The listing builds one solid part. Answer for the finished solid, in the listing's coordinates (mm). Round coordinates to 2 decimals unless told otherwise and drop trailing zeros. Loops run counter-clockwise (first coordinate to the right, second up) from the corner with the lowest first, then second, coordinate; pieces in that order, holes last. Notation, with made-up numbers: (78.25, 40.5) -> (120.25, 40.5) arc R21 cw to (120.25, 51.5) -> close; hole circle Ø3 at (36, 74). An arc over 180 degrees is marked (long way). Write each question's results on one line, items separated by ' | '. Start each with the question number.
(1) The part is cut by section A-A (x = 63). Determine the outline of the cut face in (y, z), plus the area to 3 significant figures.
(2) Flat-ended cylindrical pins translate along their axes: pin 1 (0.9 mm diameter, centred on x = 118.5, y = 1.5, fed in from -Z); pin 2 (1.5 mm diameter, centred on x = 118, y = 2, fed in from +Z); pin 3 (1.5 mm diameter, centred on x = 118, y = 1.5, fed in from -Z). Find the tip coordinate at first contact, or state that the pin passes through.
(3) The part is cut by section B-B (z = -28). Determine the outline of the cut face in (x, y).
(4) The part is cut by section C-C (x = 102.5). Determine the outline of the cut face in (y, z).
(5) The part is cut by section D-D (y = 1.45). Count the separate pieces of the cut face and the enclosed holes in it, plus the area to 3 significant figures.
(6) Straight lines are drawn through the part: probe 1 along X at (y, z) = (1.85, -60); probe 2 along Z at (x, y) = (82.5, 2.15); probe 3 along Z at (x, y) = (67.5, 0.9). For each, find the intervals that lie inside material, in ascending order.
```python
from build123d import *

# Parameters (mm, degrees)
BOSS_EXTRUDE1_DEPTH = 3
CUT_EXTRUDE1_REACH  = 162.106
SKETCH2_W           = 45
SKETCH2_H           = 74
FILLET2_R           = 3
SKETCH3_W           = 3.1
SKETCH3_H           = 10.1
CUT_EXTRUDE2_DEPTH  = 161.106214745
CUT_EXTRUDE3_REACH  = 162.106
SKETCH4_R           = 1.6


with BuildPart() as part:
    # Sketch1 → Boss-Extrude1 (new body)
    with BuildSketch(Plane(origin=(0, 0, 0), x_dir=(1, 0, 0), z_dir=(0, 1, 0))):
        Polygon((42.5, 100), (85, 100), (125, 76.905989232), (125, -76.905989232), (85, -100), (42.5, -100), align=None)
        with BuildLine():
            Line((99.3, 23), (67.3, 23))
            ThreePointArc((67.3, 23), (63.764466094, 21.535533906), (62.3, 18))
            Line((62.3, 18), (62.3, -14))
            ThreePointArc((62.3, -14), (63.764466094, -17.535533906), (67.3, -19))
            Line((67.3, -19), (99.3, -19))
            ThreePointArc((99.3, -19), (102.835533906, -17.535533906), (104.3, -14))
            Line((104.3, -14), (104.3, 18))
            ThreePointArc((104.3, 18), (102.835533906, 21.535533906), (99.3, 23))
        make_face(mode=Mode.SUBTRACT)
    extrude(amount=BOSS_EXTRUDE1_DEPTH)

    # Sketch2 → Cut-Extrude1 (cut, up to next)
    with BuildSketch(Plane(origin=(0, 3, 0), x_dir=(1, 0, 0), z_dir=(0, 1, 0)), mode=Mode.PRIVATE) as cut_extrude1_sk1:
        with Locations((65, 18)):
            Rectangle(SKETCH2_W, SKETCH2_H)
    cut_extrude1_tool1 = extrude(cut_extrude1_sk1.sketch, amount=-CUT_EXTRUDE1_REACH, mode=Mode.PRIVATE) & part.part
    add(cut_extrude1_tool1.solids().sort_by_distance((65, 3, -18))[0], mode=Mode.SUBTRACT)

    # Fillet2
    fillet2_edges = [part.edges().sort_by_distance(p)[0] for p in [
        (125, 1.5, -76.905989232),
        (125, 1.5, 76.905989232),
        (85, 1.5, 100),
        (42.5, 1.5, 100),
        (42.5, 1.5, -100),
        (85, 1.5, -100),
        (42.5, 1.5, 19),
        (42.5, 1.5, -55),
        (87.5, 1.5, -23),
        (87.5, 1.5, -55),
    ]]
    fillet(fillet2_edges, radius=FILLET2_R)

    # Sketch3 → Cut-Extrude2 (cut, through all)
    with BuildSketch(Plane(origin=(0, 3, 0), x_dir=(1, 0, 0), z_dir=(0, 1, 0))):
        with Locations((118.45, 20)):
            Rectangle(SKETCH3_W, SKETCH3_H)
        with Locations((118.45, -20)):
            Rectangle(SKETCH3_W, SKETCH3_H)
        with Locations((118.45, 60)):
            Rectangle(SKETCH3_W, SKETCH3_H)
        with Locations((118.45, -60)):
            Rectangle(SKETCH3_W, SKETCH3_H)
    extrude(amount=-CUT_EXTRUDE2_DEPTH, mode=Mode.SUBTRACT)

    # Sketch4 → Cut-Extrude3 (cut, up to next)
    with BuildSketch(Plane(origin=(0, 3, 0), x_dir=(1, 0, 0), z_dir=(0, 1, 0)), mode=Mode.PRIVATE) as cut_extrude3_sk1:
        with Locations(Location((50.5, 92, 0), (0, 0, 270))):
            Circle(SKETCH4_R)
    cut_extrude3_tool1 = extrude(cut_extrude3_sk1.sketch, amount=-CUT_EXTRUDE3_REACH, mode=Mode.PRIVATE) & part.part
    # Sketch4 → Cut-Extrude3 (cut, up to next)
    with BuildSketch(Plane(origin=(0, 3, 0), x_dir=(1, 0, 0), z_dir=(0, 1, 0)), mode=Mode.PRIVATE) as cut_extrude3_sk2:
        with Locations(Location((47.5, 60, 0), (0, 0, 270))):
            Circle(SKETCH4_R)
    cut_extrude3_tool2 = extrude(cut_extrude3_sk2.sketch, amount=-CUT_EXTRUDE3_REACH, mode=Mode.PRIVATE) & part.part
    # Sketch4 → Cut-Extrude3 (cut, up to next)
    with BuildSketch(Plane(origin=(0, 3, 0), x_dir=(1, 0, 0), z_dir=(0, 1, 0)), mode=Mode.PRIVATE) as cut_extrude3_sk3:
        with Locations(Location((47.5, -60, 0), (0, 0, 270))):
            Circle(SKETCH4_R)
    cut_extrude3_tool3 = extrude(cut_extrude3_sk3.sketch, amount=-CUT_EXTRUDE3_REACH, mode=Mode.PRIVATE) & part.part
    # Sketch4 → Cut-Extrude3 (cut, up to next)
    with BuildSketch(Plane(origin=(0, 3, 0), x_dir=(1, 0, 0), z_dir=(0, 1, 0)), mode=Mode.PRIVATE) as cut_extrude3_sk4:
        with Locations(Location((50.5, -92, 0), (0, 0, 270))):
            Circle(SKETCH4_R)
    cut_extrude3_tool4 = extrude(cut_extrude3_sk4.sketch, amount=-CUT_EXTRUDE3_REACH, mode=Mode.PRIVATE) & part.part
    # Sketch4 → Cut-Extrude3 (cut, up to next)
    with BuildSketch(Plane(origin=(0, 3, 0), x_dir=(1, 0, 0), z_dir=(0, 1, 0)), mode=Mode.PRIVATE) as cut_extrude3_sk5:
        with Locations(Location((117, 72.287187079, 0), (0, 0, 270))):
            Circle(SKETCH4_R)
    cut_extrude3_tool5 = extrude(cut_extrude3_sk5.sketch, amount=-CUT_EXTRUDE3_REACH, mode=Mode.PRIVATE) & part.part
    # Sketch4 → Cut-Extrude3 (cut, up to next)
    with BuildSketch(Plane(origin=(0, 3, 0), x_dir=(1, 0, 0), z_dir=(0, 1, 0)), mode=Mode.PRIVATE) as cut_extrude3_sk6:
        with Locations(Location((117, -72.287187079, 0), (0, 0, 270))):
            Circle(SKETCH4_R)
    cut_extrude3_tool6 = extrude(cut_extrude3_sk6.sketch, amount=-CUT_EXTRUDE3_REACH, mode=Mode.PRIVATE) & part.part
    # Sketch4 → Cut-Extrude3 (cut, up to next)
    with BuildSketch(Plane(origin=(0, 3, 0), x_dir=(1, 0, 0), z_dir=(0, 1, 0)), mode=Mode.PRIVATE) as cut_extrude3_sk7:
        with Locations(Location((82.856406461, 92, 0), (0, 0, 270))):
            Circle(SKETCH4_R)
    cut_extrude3_tool7 = extrude(cut_extrude3_sk7.sketch, amount=-CUT_EXTRUDE3_REACH, mode=Mode.PRIVATE) & part.part
    # Sketch4 → Cut-Extrude3 (cut, up to next)
    with BuildSketch(Plane(origin=(0, 3, 0), x_dir=(1, 0, 0), z_dir=(0, 1, 0)), mode=Mode.PRIVATE) as cut_extrude3_sk8:
        with Locations(Location((82.856406461, -92, 0), (0, 0, 270))):
            Circle(SKETCH4_R)
    cut_extrude3_tool8 = extrude(cut_extrude3_sk8.sketch, amount=-CUT_EXTRUDE3_REACH, mode=Mode.PRIVATE) & part.part
    add(cut_extrude3_tool1.solids().sort_by_distance((50.5, 3, -92))[0], mode=Mode.SUBTRACT)
    add(cut_extrude3_tool2.solids().sort_by_distance((47.5, 3, -60))[0], mode=Mode.SUBTRACT)
    add(cut_extrude3_tool3.solids().sort_by_distance((47.5, 3, 60))[0], mode=Mode.SUBTRACT)
    add(cut_extrude3_tool4.solids().sort_by_distance((50.5, 3, 92))[0], mode=Mode.SUBTRACT)
    add(cut_extrude3_tool5.solids().sort_by_distance((117, 3, -72.287187))[0], mode=Mode.SUBTRACT)
    add(cut_extrude3_tool6.solids().sort_by_distance((117, 3, 72.287187))[0], mode=Mode.SUBTRACT)
    add(cut_extrude3_tool7.solids().sort_by_distance((82.856406, 3, -92))[0], mode=Mode.SUBTRACT)
    add(cut_extrude3_tool8.solids().sort_by_distance((82.856406, 3, 92))[0], mode=Mode.SUBTRACT)


solid = part.part
```
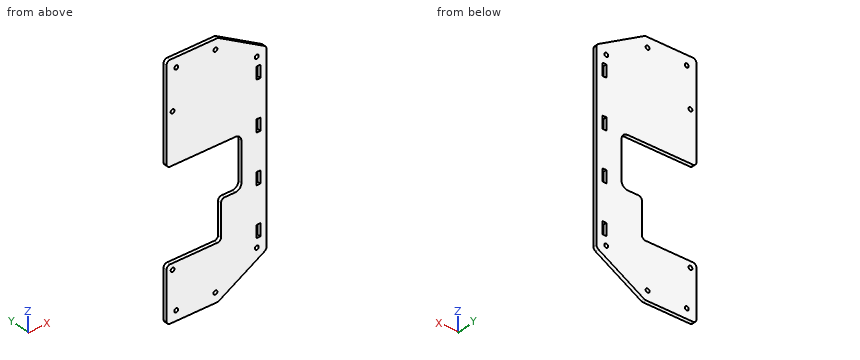
Checked values:
1) outline: (0, -100) -> (3, -100) -> (3, -55) -> (0, -55) -> close; (0, 19) -> (3, 19) -> (3, 100) -> (0, 100) -> close | area: 378 mm2
2) pin 1: stops at z = -80.92 | pin 2: stops at z = 81.38 | pin 3: stops at z = -81.38
3) outline: (87.5, 0) -> (125, 0) -> (125, 3) -> (87.5, 3) -> close
4) outline: (0, -89.9) -> (3, -89.9) -> (3, -21.84) -> (0, -21.84) -> close; (0, 17.84) -> (3, 17.84) -> (3, 89.9) -> (0, 89.9) -> close
5) separate pieces: 1 | enclosed holes: 12 | area: 11,400 mm2
6) probe 1: x = 42.5 to 45.9, 49.1 to 116.9, 120 to 125 | probe 2: z = -100 to -93.56, -90.44 to -55, 19 to 90.44, 93.56 to 100 | probe 3: z = -100 to -55, 19 to 100
